Can you work these out from the model? Positions are in its coordinate system, mm. A direction names the side the tool comes from. Round coordinates to 2 decimals unless told otherwise and drop trailing zeros. Order: outer loops, then holes, each group sorted by start corner. A loop starts at its lowest first (then second) coordinate and runs counter-clockwise, first axis right, second up. Notation, with made-up numbers: M 6,80 L 30,80 A22 cw 30,94 Z; hole C -17.5,71.25 d4. An arc over 180 degrees is marked long. One line per question, with ' | ' between items.
Autodesk Fusion 360 part; units mm, degrees
sketch "Szkic1" plane through (0, 0, 0) normal (0, 0, 1) x (1, 0, 0)
  line L0 (29, -30) -> (29, 10)
  line L1 (-31, -30) -> (29, -30)
  line L2 (-31, 10) -> (-31, -30)
  line L3 (29, 10) -> (-31, 10)
  line L4 (-10, -1) -> (10, -1)
  line L5 (-10, -25) -> (-10, -1)
  line L6 (10, -25) -> (-10, -25)
  line L7 (10, -1) -> (10, -25)
  circle A0 centre (15, -20) radius 2
  circle A1 centre (15, 0) radius 2
  circle A2 centre (-20, 0) radius 2
  circle A3 centre (-20, -20) radius 2
  line L8 (29, 10) -> (29, -30)
  line L9 (29, -30) -> (35, -30)
  line L10 (35, -30) -> (35, 10)
  line L11 (35, 10) -> (29, 10)
  line L12 (-31, 10) -> (-31, -30)
  line L13 (-31, -30) -> (-45, -30)
  line L14 (-45, -30) -> (-45, 10)
  line L15 (-45, 10) -> (-31, 10)
  line L16 (35, -30) -> (35, -260)
  line L17 (-45, -30) -> (-45, -260)
  line L18 (-45, -260) -> (35, -260)
  circle A4 centre (-20, 0) radius 3.5
  circle A5 centre (-20, -20) radius 3.5
  circle A6 centre (15, -20) radius 3.5
  circle A7 centre (15, 0) radius 3.5
  dimension "d1" = 4
  dimension "d2" = 4
  dimension "d3" = 4
  dimension "d4" = 6
  dimension "d5" = 14
  dimension "d6" = 230
  dimension "d7" = 230
  dimension "d8" = 7
  dimension "d9" = 7
  dimension "d10" = 7
  dimension "d11" = 7
extrude "Wyciągnięcie proste1" add sketch "Szkic1" against normal blind 10 contours L0 L1 L2 L3 L8 L12 | L1 L9 L13 L16 L17 L18 | L2 L12 L13 L14 L15 | A4 | A5 | A6 | A7
extrude "Wyciągnięcie proste2" cut sketch "Szkic1" against normal blind 5 contours A4 | A5 | A6 | A7
sketch "Szkic2" plane through (0, 0, -10) normal (0, 0, -1) x (1, 0, 0)
  circle A0 centre (-20, 20) radius 2
  line L0 (10, 1) -> (-10, 1)
  line L1 (-10, 1) -> (-10, 25)
  line L2 (-10, 25) -> (10, 25)
  line L3 (10, 25) -> (10, 1)
  circle A1 centre (15, 20) radius 2
  circle A2 centre (15, 0) radius 2
  circle A3 centre (-20, 0) radius 2
  line L4 (-45, 260) -> (-45, -10)
  line L5 (-45, -10) -> (29, -10)
  line L6 (29, -10) -> (29, 30)
  line L7 (29, 30) -> (35, 30)
  line L8 (35, 30) -> (35, 260)
  line L9 (35, 260) -> (-45, 260)
  circle A4 centre (25, 250) radius 1.75
  circle A5 centre (-25, 250) radius 1.75
  circle A6 centre (25, 200) radius 1.75
  circle A7 centre (25, 150) radius 1.75
  circle A8 centre (25, 100) radius 1.75
  circle A9 centre (25, 50) radius 1.75
  circle A10 centre (25, 50) radius 3.5
  circle A11 centre (25, 100) radius 3.5
  circle A12 centre (25, 150) radius 3.5
  circle A13 centre (25, 200) radius 3.5
  circle A14 centre (25, 250) radius 3.5
  circle A15 centre (-25, 250) radius 3.5
  dimension "d16" = 3.5
  dimension "d17" = 3.5
  dimension "d18" = 3.5
  dimension "d19" = 3.5
  dimension "d20" = 3.5
  dimension "d21" = 3.5
  dimension "d22" = 7
  dimension "d23" = 7
  dimension "d24" = 7
  dimension "d25" = 7
  dimension "d26" = 7
  dimension "d27" = 7
extrude "Wyciągnięcie proste3" cut sketch "Szkic2" against normal blind 5 contours A10 | A11 | A12 | A13 | A14 | A15
extrude "Wyciągnięcie proste4" cut 6 faces at (-25.7416, -250.3286, -10) (24.2584, -250.3286, -10) (23.7552, -199.6385, -10) (23.7552, -149.6385, -10) (25.3956, -99.1189, -10) (25.1298, -50.5687, -10) along direction (0, 0, 1) blind 10
(1) Thinking about a two-plate mould opening in Y: for faces 1 (the flat face through (-7, 10, -5)), 2 (the flat face through (29, -10, -5)), 3 (the flat face through (0, -1, -5)), which applies, released by +Y, released by -Y, zero draft, split by the parting line, or undercut?
Final values:
face 1: released by +Y | face 2: zero draft | face 3: undercut
(2) If we section it at B-B on x = 5: Please give me the cut outline in (y, z).
Final values:
outline: M -260,-10 L -25,-10 L -25,0 L -260,0 Z; M -1,-10 L 10,-10 L 10,0 L -1,0 Z
(3) Will these pins go through, and if not, where does the flat tip stop? pin 1 Ø4.5 at (x, y) = (15, 0) entering from +Z; pin 2 Ø3 at (x, y) = (25, -50) entering from +Z; pin 3 Ø6.5 at (x, y) = (-20, -20) entering from -Z; pin 4 Ø5.5 at (x, y) = (25, -200) entering from -Z.
Final values:
pin 1: z = -5 | pin 2: through | pin 3: z = -10 | pin 4: z = -5
(4) Please list where these lines run through material, in increasing order: probe 1 along Y at (x, z) = (15, -6.65); probe 2 along Y at (x, z) = (25, -1.45); probe 3 along Y at (x, z) = (15.5, -3.75). Write a range as [from, to].
Final values:
probe 1: [-260, -22], [-18, -2], [2, 10] | probe 2: [-260, -251.75], [-248.25, -201.75], [-198.25, -151.75], [-148.25, -101.75], [-98.25, -51.75], [-48.25, 10] | probe 3: [-260, -23.46], [-16.54, -3.46], [3.46, 10]
(5) If we section it at A-A on z = -3: State how many separate pieces and enclosed holes the cut face has, plus the area to 3 significant figures.
Final values:
separate pieces: 1 | enclosed holes: 11 | area: 20,700 mm^2
(6) On a 3-axis mill with a long thin cutter (end or side, diameter ignored), from which of +Z, -Z, +X, -X, +Y, -Y can I reach the whole of each face in a straight line? I mean faces 4 (the cylindrical face through (-16.66, 1.05, -2.46)), 5 (the flat face through (10, -13, -5)), 6 (the flat face through (23, -149, -5)). Say none if no direction works.
Final values:
face 4: +Z | face 5: +Z, -Z | face 6: -Z
